Design review of the part built by this model. Coordinates are the model's own, in mm. Face numbers are marked on the shaded views. A direction names the side the tool comes from. Give positions to 0.01 mm unless a question says otherwise; leave off trailing zeros. Loops run counter-clockwise (first coordinate to the right, second up) from the corner with the lowest first, then second, coordinate; pieces in that order, holes last. Notation, with made-up numbers: (40.5, 60) -> (74.5, 60) arc R22 ccw to (74.5, 87) -> close; hole circle Ø4 at (63, 78.25). An arc over 180 degrees is marked (long way). Answer in a Markdown table with one row per item. Add a question column.
(1) Consider section B-B on z = -8.5. Write out the cut boundary in (x, y).
(2) Consider section C-C on y = 7.5. Write out the cut boundary in (x, z), then the cut area to 3 significant figures.
(3) For pin 1 (3.5 mm diameter, centred on y = 6.5, z = -4.5, fed in from -X); pin 2 (4 mm diameter, centred on y = 7, z = -6, fed in from -X); pin 3 (3 mm diameter, centred on x = -3, y = 6, fed in from +Z), all flat-tipped, find the tip position at first contact; note any pin that passes through.
(4) Consider section D-D on x = -0.75. Write out the cut boundary in (y, z), then the cut area to 3 significant figures.
(5) For line 1 (X direction, y = 6.5, z = -7); line 2 (Y direction, x = -4, z = -4.5); line 3 (Z direction, x = 2, y = 7), list the stretches that pass through material, from the lowest coordinate up.
(6) For the marked faces 1, 2 and 3, list the 3-axis set-ups (+Z, -Z, +X, -X, +Y, -Y) from which the entire face can be reached by the end or side of a thin tool; tool diameter is ignored.
(7) Consider section A-A on x = -3.5. Write out the cut boundary in (y, z).
from build123d import *

# Parameters (mm, degrees)
SKETCH2_W           = 9.8
SKETCH2_H           = 9.8
BOSS_EXTRUDE1_DEPTH = 9.8
SKETCH3_W           = 5.8
SKETCH3_H           = 5.8
BOSS_EXTRUDE2_DEPTH = 4
FILLET3_R           = 1
FILLET4_R           = 0.5


with BuildPart() as part:
    # Sketch2 → Boss-Extrude1 (new body)
    with BuildSketch(Plane.XY):
        Rectangle(SKETCH2_W, SKETCH2_H)
    extrude(amount=-BOSS_EXTRUDE1_DEPTH)

    # Sketch3 → Boss-Extrude2 (add)
    with BuildSketch(Plane(origin=(0, 4.9, 0), x_dir=(1, 0, 0), z_dir=(0, 1, 0))):
        with Locations((0, 4.9)):
            Rectangle(SKETCH3_W, SKETCH3_H)
    extrude(amount=BOSS_EXTRUDE2_DEPTH)

    # Fillet3
    fillet3_edges = [part.edges().sort_by_distance(p)[0] for p in [
        (2.9, 8.9, -4.9),
        (0, 8.9, -7.8),
        (-2.9, 8.9, -4.9),
        (0, 8.9, -2),
    ]]
    fillet(fillet3_edges, radius=FILLET3_R)

    # Fillet4
    fillet4_edges = [part.edges().sort_by_distance(p)[0] for p in [
        (-4.9, 0, -9.8),
        (0, -4.9, -9.8),
        (4.9, 0, -9.8),
        (0, -4.9, 0),
        (-4.9, 0, 0),
        (0, 4.9, 0),
        (4.9, 0, 0),
        (4.9, -4.9, -4.9),
        (-4.9, -4.9, -4.9),
        (-4.9, 4.9, -4.9),
        (4.9, 4.9, -4.9),
        (0, 4.9, -9.8),
    ]]
    fillet(fillet4_edges, radius=FILLET4_R)


solid = part.part
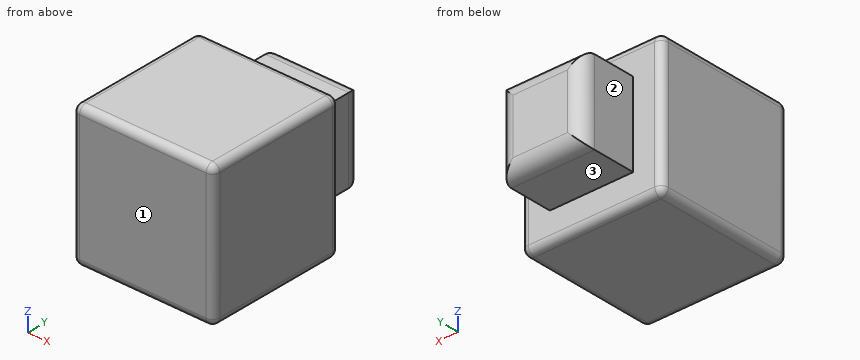
Values follow:
| question | item | result |
|---|---|---|
| 1 | outline | (-4.9, -4.4) arc R0.5 ccw to (-4.4, -4.9) -> (4.4, -4.9) arc R0.5 ccw to (4.9, -4.4) -> (4.9, 4.4) arc R0.5 ccw to (4.4, 4.9) -> (-4.4, 4.9) arc R0.5 ccw to (-4.9, 4.4) -> close |
| 2 | outline | (-2.9, -7.8) -> (2.9, -7.8) -> (2.9, -2) -> (-2.9, -2) -> close |
| 2 | area | 33.6 mm2 |
| 3 | pin 1 | x = -4.76 |
| 3 | pin 2 | x = -2.9 |
| 3 | pin 3 | z = -0.01 |
| 4 | outline | (-4.9, -9.3) arc R0.5 ccw to (-4.4, -9.8) -> (4.4, -9.8) arc R0.5 ccw to (4.9, -9.3) -> (4.9, -7.8) -> (7.9, -7.8) arc R1 ccw to (8.9, -6.8) -> (8.9, -3) arc R1 ccw to (7.9, -2) -> (4.9, -2) -> (4.9, -0.5) arc R0.5 ccw to (4.4, 0) -> (-4.4, 0) arc R0.5 ccw to (-4.9, -0.5) -> close |
| 4 | area | 119 mm2 |
| 5 | line 1 | -2.9 to 2.9 |
| 5 | line 2 | -4.9 to 4.9 |
| 5 | line 3 | -7.8 to -2 |
| 6 | face 1 | +Z, -Z, +X, -X, -Y |
| 6 | face 2 | +Z, -Z, -X, +Y |
| 6 | face 3 | -Z, +X, -X, +Y |
| 7 | outline | (-4.9, -9.3) arc R0.5 ccw to (-4.4, -9.8) -> (4.4, -9.8) arc R0.5 ccw to (4.9, -9.3) -> (4.9, -0.5) arc R0.5 ccw to (4.4, 0) -> (-4.4, 0) arc R0.5 ccw to (-4.9, -0.5) -> close |
